The model under review builds one solid part; all positions refer to its coordinate system, in mm. Round coordinates to 2 decimals unless told otherwise and drop trailing zeros. Loops run counter-clockwise (first coordinate to the right, second up) from the corner with the lowest first, then second, coordinate; pieces in that order, holes last. Notation, with made-up numbers: M 86.5,57.5 L 108.5,57.5 A18 cw 108.5,70.5 Z; hole C 83,44.5 d4. An arc over 180 degrees is marked long. Answer in a Markdown table with one row per item. Add a question column.
from build123d import *

# Parameters (mm, degrees)
F0_W     = 24.13
F0_H     = 43.18
F1_DEPTH = 0.635
F0_W_2   = 17.78
F0_H_2   = 1.27
F2_DEPTH = 1.27


with BuildPart() as f1:
    # F0 (on Top) → F1 (new body)
    with BuildSketch(Plane.XY):
        Rectangle(F0_W, F0_H)
        Polygon((8.89, -0.635), (9.525, -0.635), (9.525, -19.685), (-9.525, -19.685), (-9.525, -0.635), (-8.89, -0.635), (-8.89, 0.635), (-9.525, 0.635), (-9.525, 19.685), (9.525, 19.685), (9.525, 0.635), (8.89, 0.635), align=None, mode=Mode.SUBTRACT)
    extrude(amount=F1_DEPTH)

    # F0 (on Top) → F2 (join)
    with BuildSketch(Plane.XY):
        Rectangle(F0_W_2, F0_H_2)
    extrude(amount=F2_DEPTH)


solid = f1.part
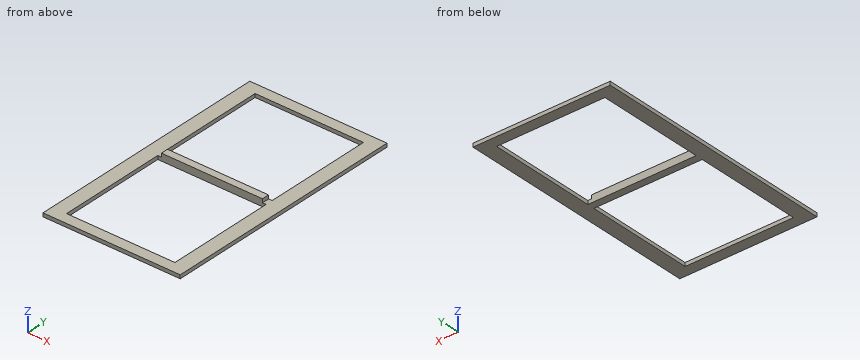
1. Take a section at C-C, the plane z = 0.85. State the section outline as (x, y) points (3 decimals), and give its area (3 significant figures).
2. Take a section at A-A, the plane y = -5.5. State the section outline as (x, z) points (3 decimals).
3. Take a section at B-B, the plane x = 8. State the section outline as (y, z) points (3 decimals), and give its area (3 significant figures).
4. To check wall thickness, follow probe 1 along Y at (x, z) = (9.25, 0.15) (3 decimals); probe 2 along X at (y, z) = (-4, 0.35) (3 decimals); probe 3 along Y at (x, z) = (7, 1.15) (3 decimals). State the ranges of each line that lie inside material, in increasing order.
5. Take a section at D-D, the plane x = -10.25. State the section outline as (y, z) points (3 decimals).
Check sheet entries:
| question | item | result |
|---|---|---|
| 1 | outline | M -8.89,-0.635 L 8.89,-0.635 L 8.89,0.635 L -8.89,0.635 Z |
| 1 | area | 22.6 mm^2 |
| 2 | outline | M -12.065,0 L -9.525,0 L -9.525,0.635 L -12.065,0.635 Z; M 9.525,0 L 12.065,0 L 12.065,0.635 L 9.525,0.635 Z |
| 3 | outline | M -21.59,0 L -19.685,0 L -19.685,0.635 L -21.59,0.635 Z; M -0.635,0 L 0.635,0 L 0.635,1.27 L -0.635,1.27 Z; M 19.685,0 L 21.59,0 L 21.59,0.635 L 19.685,0.635 Z |
| 3 | area | 4.03 mm^2 |
| 4 | probe 1 | y = -21.59 to -19.685, -0.635 to 0.635, 19.685 to 21.59 |
| 4 | probe 2 | x = -12.065 to -9.525, 9.525 to 12.065 |
| 4 | probe 3 | y = -0.635 to 0.635 |
| 5 | outline | M -21.59,0 L 21.59,0 L 21.59,0.635 L -21.59,0.635 Z |
